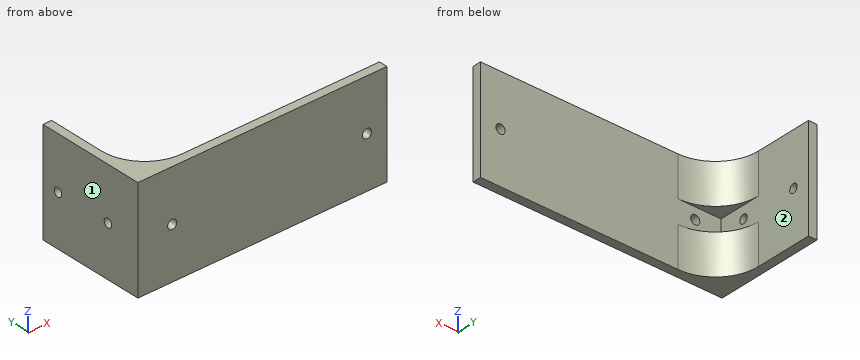
```python
from build123d import *

# Parameters (mm, degrees)
SKETCH1_W           = 87
SKETCH1_H           = 36
SKETCH1_R           = 1.6
BOSS_EXTRUDE1_DEPTH = 3
SKETCH2_W           = 3
SKETCH2_H           = 14
BOSS_EXTRUDE2_DEPTH = 35
FILLET2_R           = 15
SKETCH3_W           = 3
SKETCH3_H           = 8
BOSS_EXTRUDE3_DEPTH = 35
SKETCH4_R           = 1.5
CUT_EXTRUDE1_DEPTH  = 30


with BuildPart() as part:
    # Sketch1 → Boss-Extrude1 (new body)
    with BuildSketch(Plane(origin=(0, 0, 0), x_dir=(1, 0, 0), z_dir=(0, 1, 0))):
        with Locations((10.275590551, -4.641732283)):
            Rectangle(SKETCH1_W, SKETCH1_H)
        with Locations((46.775590551, -4.641732283)):
            Circle(SKETCH1_R, mode=Mode.SUBTRACT)
        with Locations((-21.224409449, -4.641732283)):
            Circle(SKETCH1_R, mode=Mode.SUBTRACT)
    extrude(amount=BOSS_EXTRUDE1_DEPTH)

    # Sketch2 → Boss-Extrude2 (add)
    with BuildSketch(Plane(origin=(0, 3, 0), x_dir=(1, 0, 0), z_dir=(0, 1, 0))):
        with Locations((-31.724409449, 6.358267717)):
            Rectangle(SKETCH2_W, SKETCH2_H)
        with Locations((-31.724409449, -15.641732283)):
            Rectangle(SKETCH2_W, SKETCH2_H)
    extrude(amount=BOSS_EXTRUDE2_DEPTH)

    # Fillet2
    fillet2_edges = [part.edges().sort_by_distance(p)[0] for p in [
        (-30.224409449, 3, -6.358267717),
        (-30.224409449, 3, 15.641732283),
    ]]
    fillet(fillet2_edges, radius=FILLET2_R)

    # Sketch3 → Boss-Extrude3 (add)
    with BuildSketch(Plane(origin=(0, 3, 0), x_dir=(1, 0, 0), z_dir=(0, 1, 0))):
        with Locations((-31.724409449, -4.641732283)):
            Rectangle(SKETCH3_W, SKETCH3_H)
    extrude(amount=BOSS_EXTRUDE3_DEPTH)

    # Sketch4 → Cut-Extrude1 (cut)
    with BuildSketch(Plane(origin=(-30.224409449, 0, 0), x_dir=(0, 0, -1), z_dir=(1, 0, 0))):
        with Locations((-4.324534662, 32)):
            Circle(SKETCH4_R)
        with Locations((-4.324534662, 12)):
            Circle(SKETCH4_R)
    extrude(amount=-CUT_EXTRUDE1_DEPTH, mode=Mode.SUBTRACT)


solid = part.part
```
Design review of the part built by this model. Coordinates are the model's own, in mm. Face numbers are marked on the shaded views. A direction names the side the tool comes from. Give positions to 0.01 mm unless a question says otherwise; leave off trailing zeros. Order: outer loops, then holes, each group sorted by start corner. A loop starts at its lowest first (then second) coordinate and runs counter-clockwise, first axis right, second up. Notation, with made-up numbers: (45, 26) - (78, 26) arc R17 cw to (78, 42) - close; hole circle Ø8 at (58, -20). An arc over 180 degrees is marked (long way). Use a Markdown table: item, result. Add a question column.
(1) Clearance check with a flat-ended pin moving along its axis: P1, Ø3, axis at x = 38, z = 3, coming from the +Y side. State where the tip first meets the part, or that it passes through.
(2) Machinability: for the marked faces 1 and 2, which of the approach directions +Z, -Z, +X, -X, +Y, -Y give a long, thin tool a straight path to every point of the face, cutting with its end or side? Answer none if there is none.
(3) Add section A-A on y = 32. Give the boundary of the cut face in (x, z), then the cut area to 3 significant figures.
(4) Add section D-D on y = 19.5. Give the boundary of the cut face in (x, z), then the cut area to 3 significant figures.
(5) Add section B-B on z = -8. Give the boundary of the cut face in (x, y).
(6) Add section C-C on x = -17.5. Give the boundary of the cut face in (y, z), then the cut area to 3 significant figures.
(7) Wall thickness on probe 1 along Y at (x, z) = (11, -8); probe 2 along X at (y, z) = (31, -3); probe 3 along X at (y, z) = (10, 17): over which ranges is each line inside the solid? List them lowest first. Write a range as [from, to].
Report:
| question | item | result |
|---|---|---|
| 1 | P1 | stops at y = 3 |
| 2 | face 1 | +Z, -Z, -X, +Y, -Y |
| 2 | face 2 | +X, +Y |
| 3 | outline | (-33.22, -13.36) - (-30.22, -13.36) - (-30.22, 2.82) - (-33.22, 2.82) - close; (-33.22, 5.82) - (-30.22, 5.82) - (-30.22, 22.64) - (-33.22, 22.64) - close |
| 3 | area | 99.0 mm² |
| 4 | outline | (-33.22, -13.36) - (-30.22, -13.36) - (-30.22, 22.64) - (-33.22, 22.64) - close |
| 4 | area | 108 mm² |
| 5 | outline | (-33.22, 0) - (53.78, 0) - (53.78, 3) - (-15.22, 3) arc R15 cw to (-30.22, 18) - (-30.22, 38) - (-33.22, 38) - close |
| 6 | outline | (0, -13.36) - (3.17, -13.36) - (3.17, 0.64) - (3, 0.64) - (3, 8.64) - (3.17, 8.64) - (3.17, 22.64) - (0, 22.64) - close |
| 6 | area | 113 mm² |
| 7 | probe 1 | y = [0, 3] |
| 7 | probe 2 | x = [-33.22, -30.22] |
| 7 | probe 3 | x = [-33.22, -27.91] |
